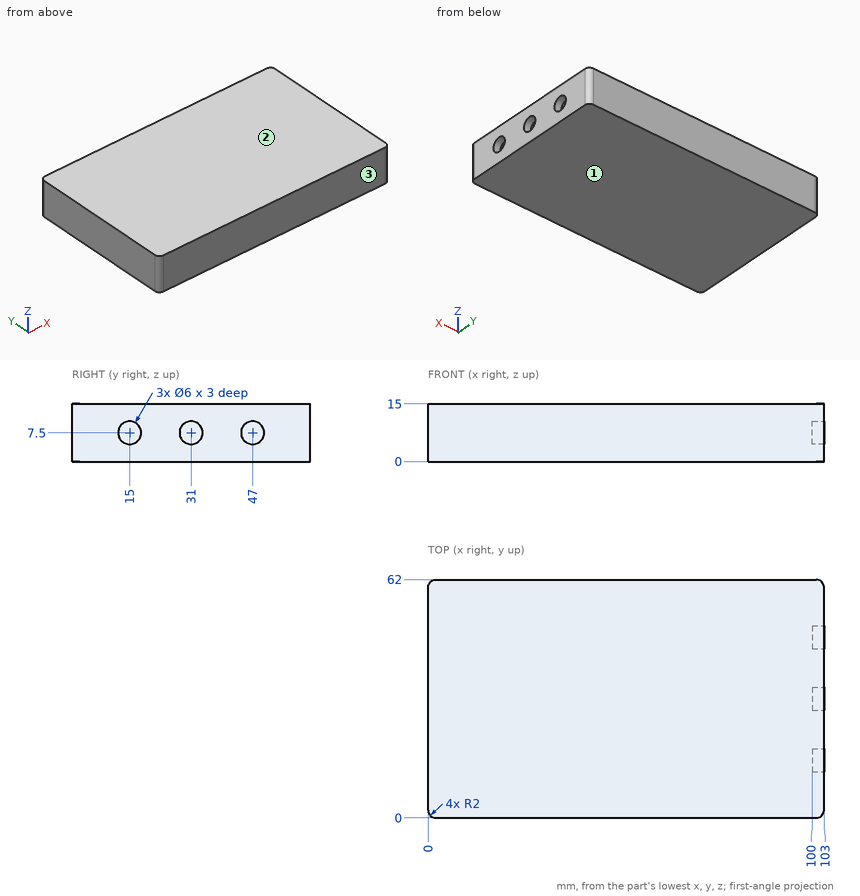
Drawing for the job (mm, zero at the part's lowest x, y, z). Round coordinates to 2 decimals unless told otherwise and drop trailing zeros. Use a Markdown table: item, result. Add a question column.
(1) Drill centre lines: line 1 (Y direction, x = 100.95, z = 7.5); line 2 (Y direction, x = 102.1, z = 7.5); line 3 (X direction, y = 17, z = 7.75). Where is each one in solid material? Low to high.
(2) Pull direction Z, two halves, no side cores. Call the marked faces 1, 2 and 3: +Z half, -Z half, draft (parallel to the pull), parting line (faces both ways), or undercut.
(3) Flat gauge pin, fed straight in: pin 1 (3 mm diameter, centred on y = 47, z = 6.5, fed in from +X). Where does the tip first touch, or does it go through?
Geometry says:
| question | item | result |
|---|---|---|
| 1 | line 1 | y = 0 to 12, 18 to 28, 34 to 44, 50 to 62 |
| 1 | line 2 | y = 0.33 to 12, 18 to 28, 34 to 44, 50 to 61.67 |
| 1 | line 3 | x = 0 to 100 |
| 2 | face 1 | -Z half |
| 2 | face 2 | +Z half |
| 2 | face 3 | draft |
| 3 | pin 1 | stops at x = 100 |
